Input: part model. Units: mm. Frame: model coordinates. Coordinates: 2 decimals unless noted, no trailing zeros. Order: outer loops, then holes, each group sorted by start corner. A loop starts at its lowest first (then second) coordinate and runs counter-clockwise, first axis right, second up. Notation, with made-up numbers: M 46.25,36.5 L 104.25,36.5 A8 cw 104.25,45.5 Z; hole C 67,-26 d3. An arc over 180 degrees is marked long. One line per item, written item: value.
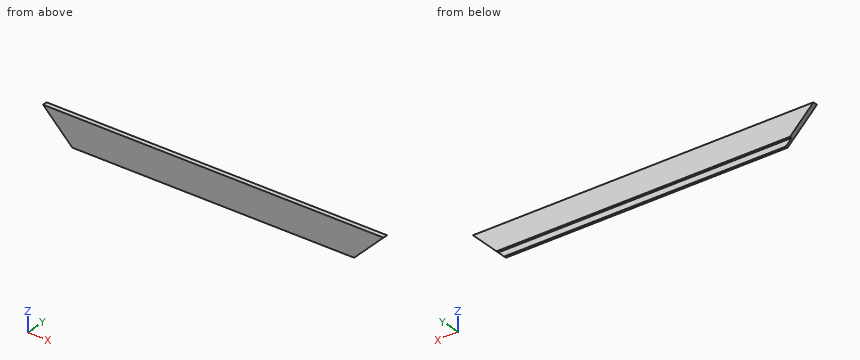
Autodesk Inventor part; units mm, degrees
ref_plane "YZ Plane" through (0, 0, 0) normal (1, 0, 0) x (0, 1, 0)
ref_plane "XZ Plane" through (0, 0, 0) normal (0, 1, 0) x (-1, 0, 0)
ref_plane "XY Plane" through (0, 0, 0) normal (0, 0, 1) x (1, 0, 0)
sketch "Sketch1" plane through (0, 0, 0) normal (1, 0, 0) x (0, 1, 0)
  line L0 (0, 0) -> (0, -127)
  line L1 (0, -127) -> (10, -127)
  line L2 (10, -127) -> (10, -101.6)
  line L3 (10, -101.6) -> (20, -101.6)
  line L4 (20, -101.6) -> (20, 0)
  line L5 (20, 0) -> (0, 0)
  dimension "d0" = 127
  dimension "d1" = 10
  dimension "d2" = 25.4
  dimension "d3" = 10
extrude "Extrusion1" add sketch "Sketch1" along normal blind 1473.2
chamfer "Chamfer1" distance 127 angle 45 1 edges at (1473.2, 5, -127)
chamfer "Chamfer2" distance 127 angle 45 1 edges at (0, 5, -127)
properties part number "SkirtLength" material "Wood (Birch)"
(1) First-contact query: pin 1 (10 mm diameter, centred on y = 14, z = -18, fed in from -X); pin 2 (4 mm diameter, centred on y = 13, z = -42, fed in from +X); pin 3 (3 mm diameter, centred on x = 628.5, y = 14, fed in from -Z). Flat tips, straight axial feed; report the tip coordinate or a pass-through.
Data:
pin 1: stops at x = 13
pin 2: stops at x = 1433.2
pin 3: stops at z = -101.6
(2) Ray query, line 1 (Z direction, x = 389, y = 11.5); line 2 (Y direction, x = 826, z = -106); line 3 (X direction, y = 9.5, z = -30). Return the intervals inside material, ascending. Write a range as from..to.
Data:
line 1: z = -101.6..0
line 2: y = 0..10
line 3: x = 30..1443.2
(3) Cut plane C-C on z = -86. Output: boundary loops of the cut face in (x, y).
Data:
outline: M 86,0 L 1387.2,0 L 1387.2,20 L 86,20 Z
(4) Cut plane D-D on z = -28.5. Output: boundary loops of the cut face in (x, y).
Data:
outline: M 28.5,0 L 1444.7,0 L 1444.7,20 L 28.5,20 Z
(5) Cut plane B-B on x = 737. Output: boundary loops of the cut face in (y, z).
Data:
outline: M 0,-127 L 10,-127 L 10,-101.6 L 20,-101.6 L 20,0 L 0,0 Z
